Here's the drawing with two shaded views (mm, measured from the low corner). I have some questions. Round coordinates to 2 decimals unless told otherwise and drop trailing zeros. Loops run counter-clockwise (first coordinate to the right, second up) from the corner with the lowest first, then second, coordinate; pieces in that order, holes last.
(1) I want a section at C-C on x = 4. Write out the boundary of the cut face in (y, z), plus the area to 3 significant figures.
(2) I want a section at B-B on z = 0.5. Write out the boundary of the cut face in (x, y).
(3) If I drill on line 1 along X through (y, z) = (4, 0.5); line 2 along X through (y, z) = (4.75, 0.45); line 3 along Y through (x, z) = (4, 0.6), over which ranges is the centre line in solid material (lowest first)?
(4) I want a section at D-D on x = 51. Write out the boundary of the cut face in (y, z).
(5) I want a section at A-A on y = 5. Write out the boundary of the cut face in (x, z), plus the area to 3 significant figures.
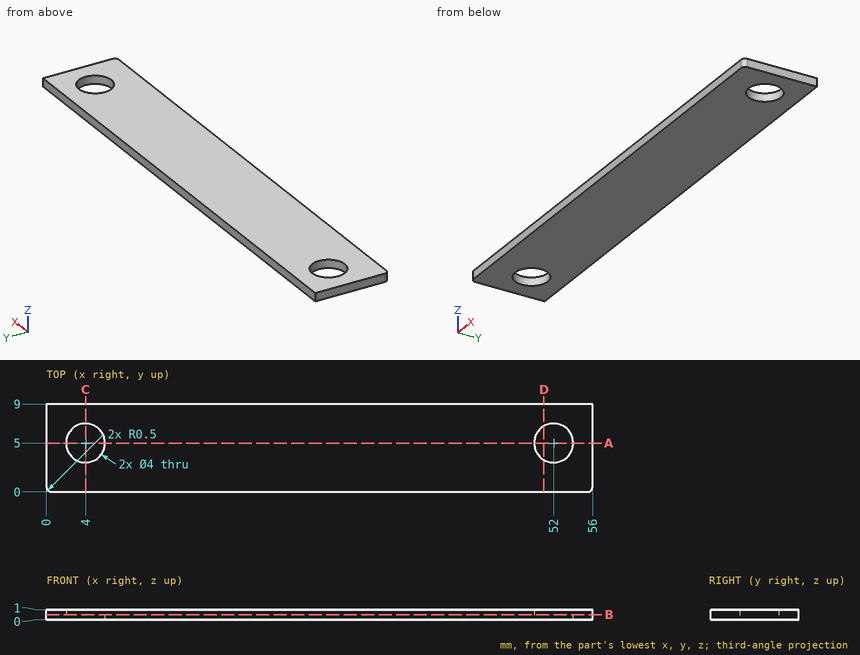
Filled sheet:
1. outline: (0, 0) - (3, 0) - (3, 1) - (0, 1) - close; (7, 0) - (9, 0) - (9, 1) - (7, 1) - close
1. area: 5.00 mm2
2. outline: (0, 0.5) arc R0.5 ccw to (0.5, 0) - (55.5, 0) arc R0.5 ccw to (56, 0.5) - (56, 9) - (0, 9) - close; hole circle Ø4 at (4, 5); hole circle Ø4 at (52, 5)
3. line 1: x = 0 to 2.27, 5.73 to 50.27, 53.73 to 56
3. line 2: x = 0 to 2.02, 5.98 to 50.02, 53.98 to 56
3. line 3: y = 0 to 3, 7 to 9
4. outline: (0, 0) - (3.27, 0) - (3.27, 1) - (0, 1) - close; (6.73, 0) - (9, 0) - (9, 1) - (6.73, 1) - close
5. outline: (0, 0) - (2, 0) - (2, 1) - (0, 1) - close; (6, 0) - (50, 0) - (50, 1) - (6, 1) - close; (54, 0) - (56, 0) - (56, 1) - (54, 1) - close
5. area: 48.0 mm2
